Could you check a few things on this drawing? It's one solid part, dimensions in mm from its lowest x, y, z. A direction names the side the tool comes from. Give positions to 0.01 mm unless a question says otherwise; leave off trailing zeros. Order: outer loops, then holes, each group sorted by start corner. A loop starts at its lowest first (then second) coordinate and runs counter-clockwise, first axis right, second up. Notation, with made-up numbers: (6.5, -32.75) -> (45.5, -32.75) arc R24 cw to (45.5, -2.75) -> close; hole circle Ø11 at (-10, 16). An arc over 180 degrees is marked (long way). Answer as CSV lines item,"result".
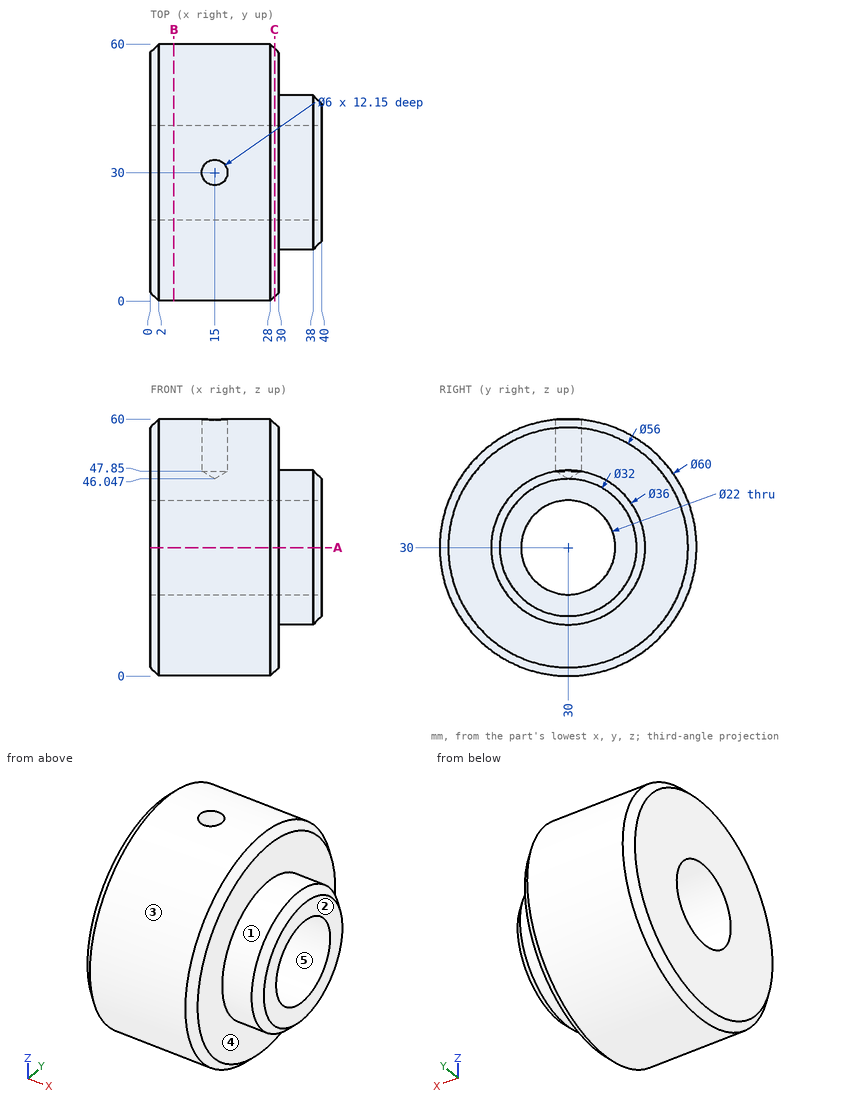
Item 1: For the marked faces 1 and 2, which set-ups out of +Z, -Z, +X, -X, +Y, -Y let a thin tool reach every point of the face, with its end or its side?
Numbers:
face 1,"+X"
face 2,"+Z, -Z, +X, +Y, -Y"
Item 2: For pin 1 (10 mm diameter, centred on x = 28.5, z = 9.5, fed in from -Y); pin 2 (5 mm diameter, centred on x = 15, y = 30, fed in from +Z); pin 3 (8 mm diameter, centred on x = 26, y = 47.5, fed in from -Z), each with a flat end and sliding along its axis, tell me the tip position at first contact or that it passes through.
Numbers:
pin 1,"stops at y = 4.33"
pin 2,"stops at z = 47.55"
pin 3,"stops at z = 3.21"
Item 3: Please list where these lines run through material, in increasing order: line 1 along Y through (x, z) = (14, 30); line 2 along Z through (x, y) = (9, 29.5); line 3 along X through (y, z) = (42, 12.5).
Numbers:
line 1,"y = 0 to 19, 41 to 60"
line 2,"z = 0 to 19.01, 40.99 to 60"
line 3,"x = 0 to 30"
Item 4: We'd pull the mould along Y, two halves only. Please class the marked faces 3, 4 and 5: released by +Y, released by -Y, zero draft, split by the parting line, or undercut.
Numbers:
face 3,"split by the parting line"
face 4,"zero draft"
face 5,"undercut"
Item 5: Imagine slicing it at A-A, the plane z = 30. Please give me the cut outline in (x, y), then the cut area to 3 significant figures.
Numbers:
outline,"(0, 2) -> (2, 0) -> (28, 0) -> (30, 2) -> (30, 12) -> (38, 12) -> (40, 14) -> (40, 19) -> (0, 19) -> close; (0, 41) -> (40, 41) -> (40, 46) -> (38, 48) -> (30, 48) -> (30, 58) -> (28, 60) -> (2, 60) -> (0, 58) -> close"
area,"1,270 mm²"
Item 6: Imagine slicing it at B-B, the plane x = 5.5. Please give me the cut outline in (y, z).
Numbers:
outline,"circle Ø60 at (30, 30); hole circle Ø22 at (30, 30)"
Item 7: Imagine slicing it at C-C, the plane x = 29. Please give me the cut outline in (y, z), then the cut area to 3 significant figures.
Numbers:
outline,"circle Ø58 at (30, 30); hole circle Ø22 at (30, 30)"
area,"2,260 mm²"
